Can you work these out from the drawing? Everything is in mm from the part's minimum corner. A direction names the side the tool comes from. Round coordinates to 2 decimals unless told otherwise and drop trailing zeros. Loops run counter-clockwise (first coordinate to the right, second up) from the corner with the lowest first, then second, coordinate; pieces in that order, holes last. Notation, with made-up numbers: (-16, 57.25) -> (-2, 57.25) arc R12 cw to (-2, 80.25) -> close; hole circle Ø5 at (-6.75, 59.25). An arc over 180 degrees is marked (long way). One line per item, written item: value.
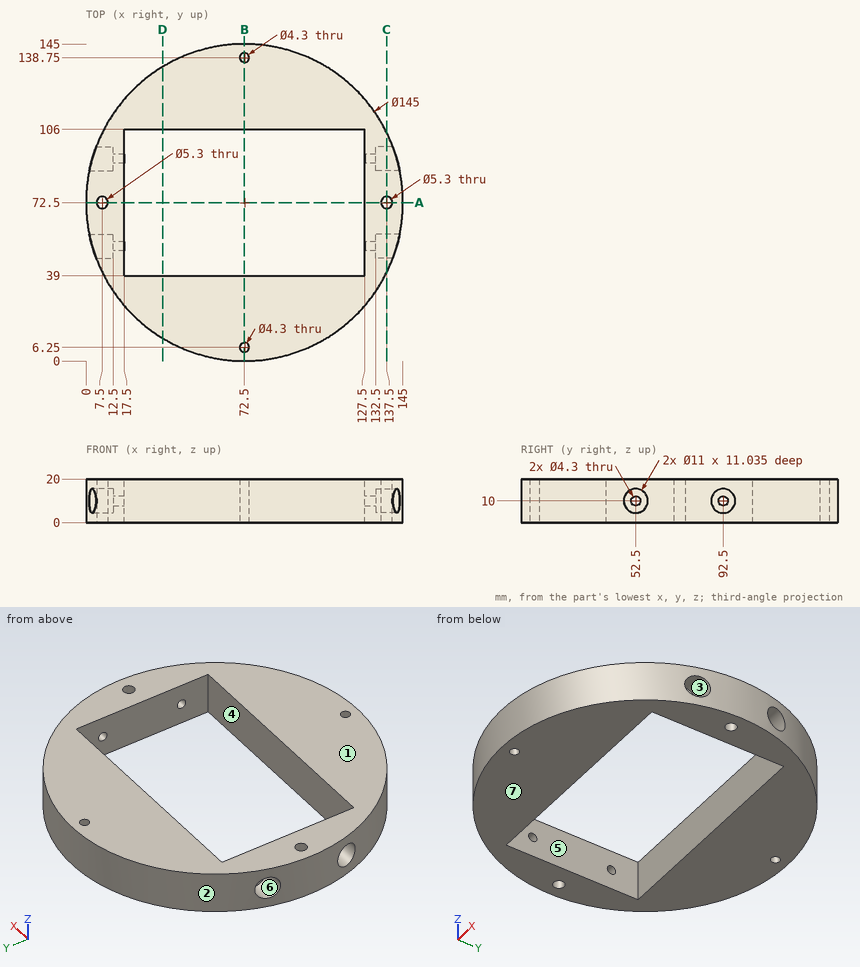
Item 1: If we section it at B-B on x = 72.5: List the corners of the cut face in (y, z) for me, plus the area to 3 significant figures.
Output:
outline: (0, 0) -> (4.1, 0) -> (4.1, 20) -> (0, 20) -> close; (8.4, 0) -> (39, 0) -> (39, 20) -> (8.4, 20) -> close; (106, 0) -> (136.6, 0) -> (136.6, 20) -> (106, 20) -> close; (140.9, 0) -> (145, 0) -> (145, 20) -> (140.9, 20) -> close
area: 1,390 mm²
Item 2: If we mould it in two halves opening along Y, with no side actions, what happens to the marked faces 1, 2, 3 and 4? For each: released by +Y, released by -Y, zero draft, split by the parting line, or undercut.
Output:
face 1: zero draft
face 2: split by the parting line
face 3: undercut
face 4: undercut
Item 3: If we section it at C-C on x = 137.5: List the corners of the cut face in (y, z) for me.
Output:
outline: (40.39, 0) -> (69.85, 0) -> (69.85, 20) -> (40.39, 20) -> close; (75.15, 0) -> (104.61, 0) -> (104.61, 20) -> (75.15, 20) -> close; hole circle Ø11 at (52.5, 10); hole circle Ø11 at (92.5, 10)
Item 4: I need wall thicknesses on line 1 (Y direction, x = 72.5, z = 7.25); line 2 (X direction, y = 89, z = 7.5); line 3 (Y direction, x = 9.75, z = 10) (1 decimal). Which ranges of each line are inside material? Lowest first, please. Write a range as from..to.
Output:
line 1: y = 0..4.1, 8.4..39, 106..136.6, 140.9..145
line 2: x = 12.5..17.5, 127.5..132.5
line 3: y = 36.2..47, 58..71.1, 73.9..87, 98..108.8
Item 5: If we section it at D-D on x = 35: List the corners of the cut face in (y, z) for me, plus the area to 3 significant figures.
Output:
outline: (10.45, 0) -> (39, 0) -> (39, 20) -> (10.45, 20) -> close; (106, 0) -> (134.55, 0) -> (134.55, 20) -> (106, 20) -> close
area: 1,140 mm²
Item 6: For the marked faces 5, 6 and 7, which set-ups out of +Z, -Z, +X, -X, +Y, -Y let a thin tool reach every point of the face, with its end or its side?
Output:
face 5: +Z, -Z
face 6: -X
face 7: -Z, +X, -X, +Y, -Y
Item 7: Will these pins go through, and if not, where does the flat tip stop? pin 1 Ø5 at (y, z) = (92.5, 10) entering from -X; pin 2 Ø6 at (y, z) = (87, 13) entering from +X; pin 3 Ø6 at (x, z) = (53, 11) entering from +Y; pin 4 Ø8.5 at (x, y) = (137.5, 72.5) entering from +Z.
Output:
pin 1: stops at x = 12.5
pin 2: stops at x = 144.08
pin 3: stops at y = 143.1
pin 4: stops at z = 20
Item 8: If we section it at A-A on y = 72.5: List the corners of the cut face in (x, z) for me.
Output:
outline: (0, 0) -> (4.85, 0) -> (4.85, 20) -> (0, 20) -> close; (10.15, 0) -> (17.5, 0) -> (17.5, 20) -> (10.15, 20) -> close; (127.5, 0) -> (134.85, 0) -> (134.85, 20) -> (127.5, 20) -> close; (140.15, 0) -> (145, 0) -> (145, 20) -> (140.15, 20) -> close
